For this review, take the finished solid that the model builds, in its own axes (mm). A direction names the side the tool comes from. Round coordinates to 2 decimals unless told otherwise and drop trailing zeros. Order: outer loops, then holes, each group sorted by start corner. A loop starts at its lowest first (then second) coordinate and runs counter-clockwise, first axis right, second up. Notation, with made-up numbers: (89.25, -2.5) -> (113.25, -2.5) arc R12 cw to (113.25, 2.5) -> close; hole circle Ø8 at (3, 58.25). An arc over 180 degrees is marked (long way). Use a Markdown table: item, result. Add a question column.
1) Clearance check with flat-ended pins moving along their axes: P1, Ø4.5, axis at y = 4, z = 6, coming from the -X side; P2, Ø7, axis at x = -8, z = 10.5, coming from the +Y side; P3, Ø7, axis at x = -10, z = 7.5, coming from the -Y side. State where each tip first meets the part, or that it passes through.
2) Consider section A-A (y = 2.5). State the section outline as (x, z) points.
3) Draft analysis for pull direction Z (two halves, no side actions). For faces 1 (the face through (-16.297, -15.035, 13.859)), 2 (the face through (-16.297, -15.035, 1.141)), 3 (the face through (-12.4, -15, 5.7)), 4 (the face through (2.5, 0, 11)), state which applies: pulls with the +Z half, pulls with the -Z half, needs draft (parallel to the pull), parting line crosses it, or undercut.
4) Consider section D-D (x = -1.25). State the section outline as (y, z) points, plus the area to 3 significant figures.
5) Machinability: for faces 5 (the face through (0, 17.5, 7)), 6 (the face through (-2.5, 3, 4)), which of the approach directions +Z, -Z, +X, -X, +Y, -Y give a long, thin tool a straight path to every point of the face, cutting with its end or side? Answer none if there is none.
6) Consider section C-C (z = 7.5). State the section outline as (x, y) points.
7) Consider section B-B (x = -10). State the section outline as (y, z) points, plus the area to 3 significant figures.
8) Wall thickness on line 1 along Z through (x, y) = (-10, -16.2); line 2 along X through (y, z) = (0, 12.5); line 3 along Y through (x, z) = (-0.5, 6.75): over which ranges is each line inside the solid? List them lowest first. Write a range as [from, to].
```python
from build123d import *

# Parameters (mm, degrees)
F5_DEPTH = 15
F0_R     = 3
F1_DEPTH = 5
F7_R     = 4
F8_R     = 1
F2_R     = 1
F3_D     = 6


with BuildPart() as f5:
    # F4 (on Top) → F5 (new body)
    with BuildSketch(Plane.XY):
        Polygon((-2.5, -17.5), (2.5, -17.5), (2.5, -12.5), (2.5, 17.5), (-2.5, 17.5), (-2.5, -12.5), (-17.5, -12.5), (-17.5, -17.5), align=None)
    extrude(amount=F5_DEPTH)

    # F0 (on face) → F1 (cut)
    with BuildSketch(Plane(origin=(-2.5, 0, 0), x_dir=(0, -1, 0), z_dir=(-1, 0, 0))):
        with Locations((-2.5, 7.5)):
            Circle(F0_R)
    extrude(amount=-F1_DEPTH, mode=Mode.SUBTRACT)

    # F7
    f7_edges = [f5.edges().sort_by_distance(p)[0] for p in [
        (0, 17.5, 15),
        (0, 17.5, 0),
        (-17.5, -15, 0),
        (-17.5, -15, 15),
    ]]
    fillet(f7_edges, radius=F7_R)

    # F8
    f8_edges = [f5.edges().sort_by_distance(p)[0] for p in [
        (-2.5, -12.5, 7.5),
    ]]
    fillet(f8_edges, radius=F8_R)

    # F2
    f2_edges = [f5.edges().sort_by_distance(p)[0] for p in [
        (2.5, -17.5, 7.5),
    ]]
    fillet(f2_edges, radius=F2_R)

    # F3 (through all)
    with Locations(Plane(origin=(0, -12.5, 0), x_dir=(-1, 0, 0), z_dir=(0, 1, 0))):
        with Locations((10, 7.5)):
            Hole(F3_D / 2)


solid = f5.part
```
Results list:
| question | item | result |
|---|---|---|
| 1 | P1 | x = -2.5 |
| 1 | P2 | y = -12.5 |
| 1 | P3 | y = -17.5 |
| 2 | outline | (-2.5, 0) -> (2.5, 0) -> (2.5, 4.5) -> (-2.5, 4.5) -> close; (-2.5, 10.5) -> (2.5, 10.5) -> (2.5, 15) -> (-2.5, 15) -> close |
| 3 | face 1 | pulls with the +Z half |
| 3 | face 2 | pulls with the -Z half |
| 3 | face 3 | undercut |
| 3 | face 4 | needs draft |
| 4 | outline | (-17.5, 0) -> (13.5, 0) arc R4 ccw to (17.5, 4) -> (17.5, 11) arc R4 ccw to (13.5, 15) -> (-17.5, 15) -> close; hole circle Ø6 at (2.5, 7.5) |
| 4 | area | 490 mm2 |
| 5 | face 5 | +Z, -Z, +X, -X, +Y |
| 5 | face 6 | +Z, -Z, -X, +Y |
| 6 | outline | (-17.5, -17.5) -> (-13, -17.5) -> (-13, -12.5) -> (-17.5, -12.5) -> close; (-7, -17.5) -> (1.5, -17.5) arc R1 ccw to (2.5, -16.5) -> (2.5, -0.5) -> (-2.5, -0.5) -> (-2.5, -11.5) arc R1 cw to (-3.5, -12.5) -> (-7, -12.5) -> close; (-2.5, 5.5) -> (2.5, 5.5) -> (2.5, 17.5) -> (-2.5, 17.5) -> close |
| 7 | outline | (-17.5, 0) -> (-12.5, 0) -> (-12.5, 4.5) -> (-17.5, 4.5) -> close; (-17.5, 10.5) -> (-12.5, 10.5) -> (-12.5, 15) -> (-17.5, 15) -> close |
| 7 | area | 45.0 mm2 |
| 8 | line 1 | [0, 4.5], [10.5, 15] |
| 8 | line 2 | [-2.5, 2.5] |
| 8 | line 3 | [-17.5, -0.4], [5.4, 17.5] |
